from build123d import *

# Parameters (mm, degrees)
F0_W     = 31.75
F0_H     = 63.5
F0_W_2   = 25.4
F0_H_2   = 57.15
F1_DEPTH = 342.9
F2_R     = 1.89865
F3_DEPTH = 3.175
F4_R     = 3.3782
F5_DEPTH = 3.175


with BuildPart() as f1:
    # F0 (on Right) → F1 (new body)
    with BuildSketch(Plane.YZ):
        Rectangle(F0_W, F0_H)
        Rectangle(F0_W_2, F0_H_2, mode=Mode.SUBTRACT)
    extrude(amount=F1_DEPTH)

    # F2 (on face) → F3 (cut, through all)
    with BuildSketch(Plane(origin=(0, 0, -31.75), x_dir=(1, 0, 0), z_dir=(0, 0, -1))):
        with Locations((117.475, 0)):
            Circle(F2_R)
        with Locations((301.625, 0)):
            Circle(F2_R)
    extrude(amount=-F3_DEPTH, mode=Mode.SUBTRACT)

    # F4 (on face) → F5 (cut, through all)
    with BuildSketch(Plane.XY.offset(31.75)):
        with Locations((19.05, 0)):
            Circle(F4_R)
        with Locations((323.85, 0)):
            Circle(F4_R)
    extrude(amount=-F5_DEPTH, mode=Mode.SUBTRACT)


solid = f1.part
Read the model definition and answer for the solid it produces. Units are mm, in the model's axes. A direction names the side the tool comes from. Give positions to 0.01 mm unless a question says otherwise; leave off trailing zeros. Write each loop counter-clockwise with the first axis right and the second up, starting at its lowest first coordinate (ties: lowest second). Pieces come first, ordered by that corner, then holes. Notation, with made-up numbers: (75, 69) - (111, 69) arc R33 cw to (111, 106) - close; hole circle Ø1 at (45, 71.5). An arc over 180 degrees is marked (long way). Use CSV: the item, a comma, the result in double quotes. Start each with the question number.
Item 1: The part is cut by section B-B, the plane z = -4. Give the vertices of the cut face in (x, y) (3 decimals), and give its area (3 significant figures).
Item 2: The mould has two halves that part along Y. Classify faces 4 (the flat face through (169, 15.875, 0)), 5 (the cylindrical face through (327.072, 1.015, 30.185)), 6 (the flat face through (169, 0, 31.75)): pulls with the +Y half, pulls with the -Y half, needs draft (parallel to the pull), parting line crosses it, or undercut.
Item 3: The part is cut by section C-C, the plane x = 323.85. Give the vertices of the cut face in (y, z) (3 decimals).
Item 4: The part is cut by section A-A, the plane x = 125. Give the vertices of the cut face in (y, z) (3 decimals), and give its area (3 significant figures).
Item 5: Consider line 1 (X direction, y = 0, z = -29.95); line 2 (Y direction, x = 323.85, z = 29.6) (3 decimals); line 3 (Z direction, x = 91.5, y = 8.5) (3 decimals). Determine where each line is inside the solid, lowest interval first.
Item 6: For faces 1 (the cylindrical face through (22.171, -1.294, 30.185)), 2 (the flat face through (342.9, -13, 3)), 3 (the flat face through (169, 0, -28.575)), determine the directions among +Z, -Z, +X, -X, +Y, -Y from which every point of the face is accessible in a straight line to the end or side of a thin tool.
Item 7: A flat-ended cylindrical pin translates along its axis: P1, Ø6, axis at x = 19.05, y = 0, coming from the +Z side (3 decimals). Find the tip coordinate at first contact, or state that the pin passes through.
Taken from the geometry:
1,outline,"(0, -15.875) - (342.9, -15.875) - (342.9, -12.7) - (0, -12.7) - close; (0, 12.7) - (342.9, 12.7) - (342.9, 15.875) - (0, 15.875) - close"
1,area,"2,180 mm2"
2,face 4,"pulls with the +Y half"
2,face 5,"undercut"
2,face 6,"needs draft"
3,outline,"(-15.875, -31.75) - (15.875, -31.75) - (15.875, 31.75) - (3.378, 31.75) - (3.378, 28.575) - (12.7, 28.575) - (12.7, -28.575) - (-12.7, -28.575) - (-12.7, 28.575) - (-3.378, 28.575) - (-3.378, 31.75) - (-15.875, 31.75) - close"
4,outline,"(-15.875, -31.75) - (15.875, -31.75) - (15.875, 31.75) - (-15.875, 31.75) - close; hole (-12.7, -28.575) - (12.7, -28.575) - (12.7, 28.575) - (-12.7, 28.575) - close"
4,area,"565 mm2"
5,line 1,"0 to 115.58, 119.37 to 299.73, 303.52 to 342.9"
5,line 2,"-15.875 to -3.378, 3.378 to 15.875"
5,line 3,"-31.75 to -28.575, 28.575 to 31.75"
6,face 1,"+Z"
6,face 2,"+Z, -Z, +X, +Y, -Y"
6,face 3,"+X, -X"
7,P1,"z = -28.575"
